Build history of the part. All positions in model axes, mm. A direction names the side the tool comes from. Give positions to 0.01 mm unless a question says otherwise; leave off trailing zeros. Order: outer loops, then holes, each group sorted by start corner. A loop starts at its lowest first (then second) coordinate and runs counter-clockwise, first axis right, second up. Notation, with made-up numbers: (30.25, 72) - (44.25, 72) arc R14 ccw to (44.25, 91) - close; hole circle Ø5 at (-25, 26). An arc over 180 degrees is marked (long way). Answer in a Markdown table with one row per item.
```python
from build123d import *

# Parameters (mm, degrees)
SKETCH1_W           = 7
SKETCH1_H           = 6
BOSS_EXTRUDE1_DEPTH = 9
SKETCH2_W           = 3
SKETCH2_H           = 5
CUT_EXTRUDE1_DEPTH  = 3
CUT_EXTRUDE2_DEPTH  = 7
SKETCH4_W           = 1
SKETCH4_H           = 2
BOSS_EXTRUDE2_DEPTH = 1
CUT_EXTRUDE3_DEPTH  = 10
CUT_EXTRUDE5_DEPTH  = 4
CUT_EXTRUDE6_DEPTH  = 3


with BuildPart() as part:
    # Sketch1 → Boss-Extrude1 (new body)
    with BuildSketch(Plane.XY):
        Rectangle(SKETCH1_W, SKETCH1_H)
    extrude(amount=BOSS_EXTRUDE1_DEPTH)

    # Sketch2 → Cut-Extrude1 (cut)
    with BuildSketch(Plane(origin=(0, 3, 0), x_dir=(1, 0, 0), z_dir=(0, 1, 0))):
        with Locations((2, -3.5)):
            Rectangle(SKETCH2_W, SKETCH2_H)
    extrude(amount=-CUT_EXTRUDE1_DEPTH, mode=Mode.SUBTRACT)

    # Sketch3 → Cut-Extrude2 (cut, through all)
    with BuildSketch(Plane(origin=(0, 3, 0), x_dir=(1, 0, 0), z_dir=(0, 1, 0))):
        Polygon((3.5, -1), (2.5, -1), (2.5, -8), (-2.5, -8), (-2.5, -9), (3.5, -9), align=None)
    extrude(amount=-CUT_EXTRUDE2_DEPTH, mode=Mode.SUBTRACT)

    # Sketch4 → Boss-Extrude2 (add)
    with BuildSketch(Plane(origin=(-2.5, 0, 0), x_dir=(0, 0, -1), z_dir=(1, 0, 0))):
        with Locations((-8.5, -2)):
            Rectangle(SKETCH4_W, SKETCH4_H)
    extrude(amount=BOSS_EXTRUDE2_DEPTH)

    # Sketch5 → Cut-Extrude3 (cut, through all)
    with BuildSketch(Plane.XY.offset(9)):
        Polygon((-3.5, 1), (-1.5, 1), (-1.5, -1), (-2.5, -1), (-2.5, -3), (-3.5, -3), align=None)
    extrude(amount=-CUT_EXTRUDE3_DEPTH, mode=Mode.SUBTRACT)

    # Sketch6 → Cut-Extrude5 (cut)
    with BuildSketch(Plane(origin=(2.5, 0, 0), x_dir=(0, 0, -1), z_dir=(1, 0, 0))):
        Polygon((-3, 3), (-8, -2), (-8, 1), (-9, 1), (-9, 3), align=None)
    extrude(amount=-CUT_EXTRUDE5_DEPTH, mode=Mode.SUBTRACT)

    # Sketch8 → Cut-Extrude6 (cut, through all)
    with BuildSketch(Plane(origin=(-1.5, 0, 0), x_dir=(0, 0, -1), z_dir=(1, 0, 0))):
        Polygon((-5, 1), (-3, 3), (-9, 3), (-9, 1), align=None)
    extrude(amount=-CUT_EXTRUDE6_DEPTH, mode=Mode.SUBTRACT)


solid = part.part
```
1. Two-plate mould, pull along Y, no slides. Class faces 1 (the face through (2, 1, 1)), 2 (the face through (-1, 3, 1)), 3 (the face through (-2, -1, 5)), 4 (the face through (-3, 1, 3)): +Y half, -Y half, draft (parallel to the pull), parting line (faces both ways), or undercut.
Check result:
| item | result |
|---|---|
| face 1 | draft |
| face 2 | +Y half |
| face 3 | undercut |
| face 4 | undercut |
2. Cut at A-A on z = 4.5. Write the cut outline in (x, y).
Check result:
| item | result |
|---|---|
| outline | (-3.5, 1) - (-1.5, 1) - (-1.5, -1) - (-2.5, -1) - (-2.5, -3) - (2.5, -3) - (2.5, 0) - (0.5, 0) - (0.5, 1.5) - (-3.5, 1.5) - close |
3. Which spindle directions (+Z, -Z, +X, -X, +Y, -Y) get a long thin tool onto all of the face, cutting with end or side? Do faces 5 (the face through (0, -3, 5)), 6 (the face through (-2.5, -2, 5)), 7 (the face through (-1.5, 0, 3)), 8 (the face through (2.5, -1, 4)), 9 (the face through (0.5, 1, 3)). Say none if no direction does.
Check result:
| item | result |
|---|---|
| face 5 | +Z, -Z, +X, -X, -Y |
| face 6 | +Z, -Z, -X, -Y |
| face 7 | +Z, -Z, -X |
| face 8 | +Z, +X, +Y, -Y |
| face 9 | +Z, +X, +Y |
4. Cut at D-D on z = 2.25. Write the cut outline in (x, y), and give its area (3 significant figures).
Check result:
| item | result |
|---|---|
| outline | (-3.5, 1) - (-1.5, 1) - (-1.5, -1) - (-2.5, -1) - (-2.5, -3) - (2.5, -3) - (2.5, 0) - (0.5, 0) - (0.5, 3) - (-3.5, 3) - close |
| area | 24.0 mm² |
5. Drop flat-ended pins along their axis: P1, Ø3.5, axis at x = 2, y = 1, coming from the +Z side; P2, Ø0.8, axis at x = -2, z = 5.5, coming from the +Y side; P3, Ø3.5, axis at y = 1.5, z = 3.5, coming from the +X side. Give the stop position or say it passes through.
Check result:
| item | result |
|---|---|
| P1 | stops at z = 6.75 |
| P2 | stops at y = -1 |
| P3 | stops at x = 2.5 |
6. Probe line 1 (Y direction, x = 0.75, z = 5); line 2 (Z direction, x = 2, y = 0.5); line 3 (Y direction, x = -1.25, z = 7.5). List the from-to ranges inside material, lowest first.
Check result:
| item | result |
|---|---|
| line 1 | y = -3 to 0 |
| line 2 | z = 0 to 1 |
| line 3 | y = -3 to -1.5 |
7. Cut at B-B on y = -1.25. Write the cut outline in (x, z), and give its area (3 significant figures).
Check result:
| item | result |
|---|---|
| outline | (-2.5, 0) - (3.5, 0) - (3.5, 1) - (2.5, 1) - (2.5, 7.25) - (-1.5, 7.25) - (-1.5, 9) - (-2.5, 9) - close |
| area | 39.0 mm² |
8. Cut at C-C on x = 2. Write the cut outline in (y, z), and give its area (3 significant figures).
Check result:
| item | result |
|---|---|
| outline | (-3, 0) - (3, 0) - (3, 1) - (0, 1) - (0, 6) - (-2, 8) - (-3, 8) - close |
| area | 25.0 mm² |
